The listing builds one solid part. Answer for the finished solid, in the listing's coordinates (mm). A direction names the side the tool comes from. Coordinates: 2 decimals unless noted, no trailing zeros. Loops run counter-clockwise (first coordinate to the right, second up) from the corner with the lowest first, then second, coordinate; pieces in that order, holes last. Notation, with made-up numbers: (48, 2.5) - (65, 2.5) arc R19 ccw to (65, 29.5) - close; hole circle Ø11 at (-15, 13). An arc over 180 degrees is marked (long way). Use one line per item in the form item = value. Start each with the question number.
```python
from build123d import *

# Parameters (mm, degrees)
F0_R            = 20.6375
F0_R_2          = 2.15265
F1_DEPTH        = 12.7
F3_DEPTH        = 12.7
F4_COUNT        = 6
F4_ANGLE        = 300
F6_R            = 11.90625
F7_DEPTH        = 11.36015
F9_DEPTH        = 12.7
F9_COPIES_COUNT = 4


# Not quite as in the source:
# - a pattern or mirror of a feature is missing from the dataset's text; its kind, count and spacing are read off the source's solid


with BuildPart() as f1:
    # F0 (on Top) → F1 (new body)
    with BuildSketch(Plane.XY):
        Circle(F0_R)
        with Locations((-11.2253201513, -11.2253201513)):
            Circle(F0_R_2, mode=Mode.SUBTRACT)
        with Locations((11.2253201513, -11.2253201513)):
            Circle(F0_R_2, mode=Mode.SUBTRACT)
        with Locations((-11.2253201513, 11.2253201513)):
            Circle(F0_R_2, mode=Mode.SUBTRACT)
        with BuildLine():
            ThreePointArc((0, 11.1125), (7.8577241059, 7.8577241059), (11.1125, 0))
            ThreePointArc((11.1125, 0), (-7.8577241059, -7.8577241059), (0, 11.1125))
        make_face(mode=Mode.SUBTRACT)
        with Locations((11.2253201513, 11.2253201513)):
            Circle(F0_R_2, mode=Mode.SUBTRACT)
    extrude(amount=F1_DEPTH)

    # F2 (on face) → F3 (cut, through all)
    with BuildSketch(Plane.XY.offset(12.7)):
        with BuildLine():
            ThreePointArc((-2.8761266387, 10.7338507446), (0, 11.1125), (2.8761266387, 10.7338507446))
            Line((2.8761266387, 10.7338507446), (3.0815642558, 11.5005543693))
            ThreePointArc((3.0815642558, 11.5005543693), (0, 11.90625), (-3.0815642558, 11.5005543693))
            Line((-3.0815642558, 11.5005543693), (-2.8761266387, 10.7338507446))
        make_face()
    f3 = extrude(amount=-F3_DEPTH, mode=Mode.SUBTRACT)

    # F4: F3 ×6 about axis
    f4_axis = Axis((0, 0, 0), (0, 0, -1))
    for i in range(1, F4_COUNT):
        add(f3.rotate(f4_axis, i * F4_ANGLE / (F4_COUNT - 1)), mode=Mode.SUBTRACT)

    # F6 (on face) → F7 (cut, through all)
    with BuildSketch(Plane(origin=(0, 0, 0), x_dir=(1, 0, 0), z_dir=(0, 0, -1))):
        Circle(F6_R)
    extrude(amount=-F7_DEPTH, mode=Mode.SUBTRACT)

    # F8 (on face) → F9 (cut, through all)
    with BuildSketch(Plane(origin=(0, 0, 0), x_dir=(1, 0, 0), z_dir=(0, 0, -1))):
        with BuildLine():
            ThreePointArc((11.5039191556, -15.1842795042), (9.251826165, -14.6686177057), (7.6685282311, -12.9860608474))
            ThreePointArc((7.6685282311, -12.9860608474), (0, -15.08125), (-7.6685282311, -12.9860608474))
            ThreePointArc((-7.6685282311, -12.9860608474), (-9.251826165, -14.6686177057), (-11.5039191556, -15.1842795042))
            ThreePointArc((-11.5039191556, -15.1842795042), (0, -19.05), (11.5039191556, -15.1842795042))
        make_face()
    f9 = extrude(amount=-F9_DEPTH, mode=Mode.SUBTRACT)

    # F9_copies: F9 ×4 about axis
    f9_copies_axis = Axis((0, 0, 0), (0, 0, 1))
    for i in range(1, F9_COPIES_COUNT):
        add(f9.rotate(f9_copies_axis, i * 360 / F9_COPIES_COUNT), mode=Mode.SUBTRACT)


solid = f1.part
```
(1) For faces 4 (the face through (6, 10, 11.36)), 5 (the face through (-9, -9, 0)), 6 (the face through (-5.521, -9.644, 12.021)), determine the directions among +Z, -Z, +X, -X, +Y, -Y from which every point of the face is accessible in a straight line to the end or side of a thin tool.
(2) Determine the mould class of faces 1 (the face through (-4.474, -20.147, 6.261)), 2 (the face through (-9, -9, 12.7)), 3 (the face through (-9.17, -10.58, 6.26)) for opening direction X: +X half, -X half, draft (parallel to the pull), parting line (faces both ways), or undercut.
(3) A cutting plane is placed at B-B (y = 5). Determine the outline of the cut face in (x, z), then the cut area to 3 significant figures.
(4) A cutting plane is placed at C-C (x = -12.5). Determine the outline of the cut face in (y, z).
(5) A cutting plane is placed at A-A (x = 0). Determine the outline of the cut face in (y, z), then the cut area to 3 significant figures.
(6) A cutting plane is placed at D-D (y = -14). Determine the outline of the cut face in (x, z), then the cut area to 3 significant figures.
(7) Each of these flat-tipped pins is pushed along its axis until it touches: pin 1 Ø3 at (x, z) = (-7.5, 6) entering from +Y; pin 2 Ø1.5 at (x, y) = (-8, 16) entering from +Z; pin 3 Ø6 at (y, z) = (4, 3.5) entering from +X; pin 4 Ø0.9 at (x, y) = (11, -1) entering from -Z. Where does it stop, or does it pass through?
(8) Find the intervals of material crossed by probe 1 along Y at (x, z) = (11, 1.5); probe 2 along Y at (x, z) = (-5, 11.75); probe 3 along Y at (x, z) = (-4.5, 9.5), in increasing order. Write a range as from..to.
Evaluation:
q1.face_4 = -Z
q1.face_5 = -Z, +X, -X, +Y, -Y
q1.face_6 = +Z, -Z
q2.face_1 = parting line
q2.face_2 = draft
q2.face_3 = undercut
q3.outline = (-20.02, 0) - (-18.38, 0) - (-18.38, 12.7) - (-20.02, 12.7) - close; (-14.23, 0) - (-10.81, 0) - (-10.81, 12.7) - (-14.23, 12.7) - close; (10.81, 0) - (14.23, 0) - (14.23, 12.7) - (10.81, 12.7) - close; (18.38, 0) - (20.02, 0) - (20.02, 12.7) - (18.38, 12.7) - close
q3.area = 129 mm^2
q4.outline = (-16.42, 0) - (-12.96, 0) - (-12.96, 12.7) - (-16.42, 12.7) - close; (-9.49, 0) - (9.49, 0) - (9.49, 12.7) - (-9.49, 12.7) - close; (12.96, 0) - (16.42, 0) - (16.42, 12.7) - (12.96, 12.7) - close
q5.outline = (-20.64, 0) - (-19.05, 0) - (-19.05, 12.7) - (-20.64, 12.7) - close; (-15.08, 0) - (-11.91, 0) - (-11.91, 12.7) - (-15.08, 12.7) - close; (11.91, 0) - (15.08, 0) - (15.08, 12.7) - (11.91, 12.7) - close; (19.05, 0) - (20.64, 0) - (20.64, 12.7) - (19.05, 12.7) - close
q5.area = 121 mm^2
q6.outline = (-15.16, 0) - (-8.39, 0) - (-8.39, 12.7) - (-15.16, 12.7) - close; (-5.61, 0) - (5.61, 0) - (5.61, 12.7) - (-5.61, 12.7) - close; (8.39, 0) - (15.16, 0) - (15.16, 12.7) - (8.39, 12.7) - close
q6.area = 315 mm^2
q7.pin_1 = 19.75
q7.pin_2 = through
q7.pin_3 = 20.61
q7.pin_4 = 11.36
q8.probe_1 = -17.46..-15.55, -15.19..-13.37, -9.08..-4.56, 4.56..9.08, 13.37..15.19, 15.55..17.46
q8.probe_2 = -20.02..-18.38, -14.23..-9.92, 9.92..14.23, 18.38..20.02
q8.probe_3 = -20.14..-18.51, -14.39..-11.02, 11.02..14.39, 18.51..20.14
